Input: part model. Units: mm. Frame: model coordinates. A direction names the side the tool comes from. Give positions to 0.01 mm unless a question says otherwise; leave off trailing zeros. Write each loop counter-clockwise with the first axis right and the second up, starting at its lowest first coordinate (ties: lowest second). Pieces come first, ordered by that corner, then holes. Notation, with made-up numbers: (-14, 21) - (32, 21) arc R25 ccw to (32, 39) - close; hole circle Ø7 at (28.25, 14.25). An arc over 180 degrees is marked (long way). Use a Markdown table: item, result. Add a question column.
1. Section query C-C, the plane x = 23. Return loops of the section in (y, z), plus the area to 3 significant figures.
2. Pin query (flat end, axial travel): pin 1 (4 mm diameter, centred on x = 113, z = 5.5, fed in from +Y); pin 2 (3 mm diameter, centred on x = 126, z = 6.5, fed in from +Y). Return the tip coordinate at first contact, or that it passes through.
3. Material intervals for probe 1 along Y at (x, z) = (91, 7); probe 2 along Y at (x, z) = (109.5, 6.75), sorted ascending.
4. Section query A-A, the plane z = 7. Return loops of the section in (x, y).
5. Set-up query: faces 1 (the flat face through (125, 155, 5)), 2 (the flat face through (66, 93, 10)). Return all of +Z, -Z, +X, -X, +Y, -Y with unobstructed straight access to the full face (end or side cutting, diameter ignored); none if empty.
6. Section query B-B, the plane x = 60. Return loops of the section in (y, z), plus the area to 3 significant figures.
```python
from build123d import *

# Parameters (mm, degrees)
BOSS_EXTRU_1_DEPTH = 10
CONG_1_R           = 4


with BuildPart() as part:
    # Esquisse1 → Boss.-Extru.1 (new body)
    with BuildSketch(Plane.XY):
        Polygon((0, 183), (10, 183), (120, 155), (130, 155), (130, 0), (0, 0), align=None)
    extrude(amount=BOSS_EXTRU_1_DEPTH)

    # Congé1
    cong_1_edges = [part.edges().sort_by_distance(p)[0] for p in [
        (0, 183, 5),
    ]]
    fillet(cong_1_edges, radius=CONG_1_R)


solid = part.part
```
Result sheet:
| question | item | result |
|---|---|---|
| 1 | outline | (0, 0) - (179.69, 0) - (179.69, 10) - (0, 10) - close |
| 1 | area | 1,800 mm² |
| 2 | pin 1 | stops at y = 157.29 |
| 2 | pin 2 | stops at y = 155 |
| 3 | probe 1 | y = 0 to 162.38 |
| 3 | probe 2 | y = 0 to 157.67 |
| 4 | outline | (0, 0) - (130, 0) - (130, 155) - (120, 155) - (10, 183) - (4, 183) arc R4 ccw to (0, 179) - close |
| 5 | face 1 | +Z, -Z, +X, +Y |
| 5 | face 2 | +Z, +X, -X, +Y, -Y |
| 6 | outline | (0, 0) - (170.27, 0) - (170.27, 10) - (0, 10) - close |
| 6 | area | 1,700 mm² |
